The model under review builds one solid part; all positions refer to its coordinate system, in mm. A direction names the side the tool comes from. Coordinates: 2 decimals unless noted, no trailing zeros. Write each loop counter-clockwise with the first axis right and the second up, starting at its lowest first coordinate (ties: lowest second). Pieces come first, ordered by that corner, then holes.
1) For P1, Ø6, axis at x = 30, y = -4, coming from the +Z side; P2, Ø6, axis at y = 22.5, z = 0, coming from the +X side; P3, Ø5, axis at x = 156, z = 17, coming from the +Y side, all flat-tipped, find the tip position at first contact; note any pin that passes through.
2) Mouldability with a two-part tool opening along X and no side actions: class faces 5 (the flat face through (144.6, -13, -13)), 6 (the cylindrical face through (194, -20, 0)), 7 (the flat face through (149.6, 13, -13)) as released by +X, released by -X, zero draft, split by the parting line, or undercut.
3) Machinability: for faces 1 (the flat face through (3, 16, -5)), 2 (the cylindrical face through (203, -2.17, 9.76)), 3 (the cylindrical face through (1.986, -13.887, 10.648)), 4 (the flat face through (27, 0, -12.5)), which of the approach directions +Z, -Z, +X, -X, +Y, -Y give a long, thin tool a straight path to every point of the face, cutting with its end or side? Answer none if there is none.
4) Add section C-C, the plane x = 88.5. State the section outline as (y, z) points, then the cut area to 3 significant figures.
5) Add section A-A, the plane z = 0. Give the number of separate pieces and of enclosed holes in the cut face, then the cut area to 3 significant figures.
6) For line 1 (Y direction, x = 196, z = 0); line 2 (X direction, y = -20, z = 11); line 3 (X direction, y = -22.5, z = -11), list the stretches that pass through material, from the lowest coordinate up.
from build123d import *

# Parameters (mm, degrees)
OTW_R_GWINTOWANY_M63_D     = 5
OTW_R_GWINTOWANY_M63_DEPTH = 10
SFAZOWANIE1_SIZE           = 1
ZAOKR_GLENIE1_R            = 0.5
SFAZOWANIE2_SIZE           = 0.5
ZAOKR_GLENIE2_R            = 0.5
WYTNIJ_WYCI_GNI_CIE1_DEPTH = 5


with BuildPart() as part:
    # Szkic1 → Obrót1 (revolve)
    with BuildSketch(Plane.XY):
        Polygon((0, 0), (207.5, 0), (207.5, 10), (199.1, 10), (199.1, 30), (189.1, 30), (189.1, 17.5), (149.6, 17.5), (149.6, 25), (144.6, 25), (144.6, 17.5), (4.6, 17.5), (4.6, 16.5), (3, 16.5), (3, 17.5), (0, 17.5), align=None)
    revolve(axis=Axis((0, 0, 0), (-1, 0, 0)))

    # Otwór gwintowany M63
    with Locations(Plane(origin=(199.1, 0, 0), x_dir=(0, 0, -1), z_dir=(1, 0, 0))):
        with Locations((0, 22.5), (22.5, 0), (0, -22.5), (-22.5, 0)):
            Hole(OTW_R_GWINTOWANY_M63_D / 2, depth=OTW_R_GWINTOWANY_M63_DEPTH)

    # Sfazowanie1
    sfazowanie1_edges = [part.edges().sort_by_distance(p)[0] for p in [
        (207.5, -10, 0),
        (0, -17.5, 0),
    ]]
    chamfer(sfazowanie1_edges, length=SFAZOWANIE1_SIZE)

    # Zaokrąglenie1
    zaokr_glenie1_edges = [part.edges().sort_by_distance(p)[0] for p in [
        (189.1, -17.5, 0),
        (149.6, -17.5, 0),
        (144.6, -17.5, 0),
    ]]
    fillet(zaokr_glenie1_edges, radius=ZAOKR_GLENIE1_R)

    # Sfazowanie2
    sfazowanie2_edges = [part.edges().sort_by_distance(p)[0] for p in [
        (199.1, -30, 0),
        (189.1, -30, 0),
        (149.6, -25, 0),
        (144.6, -25, 0),
    ]]
    chamfer(sfazowanie2_edges, length=SFAZOWANIE2_SIZE)

    # Zaokrąglenie2
    zaokr_glenie2_edges = [part.edges().sort_by_distance(p)[0] for p in [
        (199.1, -10, 0),
    ]]
    fillet(zaokr_glenie2_edges, radius=ZAOKR_GLENIE2_R)

    # Szkic7 → Wytnij-wyciągnięcie1 (cut)
    with BuildSketch(Plane(origin=(0, 0, -17.5), x_dir=(-1, 0, 0), z_dir=(0, 0, -1))):
        with BuildLine():
            Line((-12.1, -5), (-42.1, -5))
            ThreePointArc((-42.1, -5), (-47.1, 0), (-42.1, 5))
            Line((-42.1, 5), (-12.1, 5))
            ThreePointArc((-12.1, 5), (-7.1, 0), (-12.1, -5))
        make_face()
    extrude(amount=-WYTNIJ_WYCI_GNI_CIE1_DEPTH, mode=Mode.SUBTRACT)


solid = part.part
Geometry results:
1. P1: stops at z = 17.47
1. P2: stops at x = 199.1
1. P3: stops at y = 9.8
2. face 5: released by -X
2. face 6: zero draft
2. face 7: undercut
3. face 1: none
3. face 2: +X
3. face 3: -X
3. face 4: -Z
4. outline: circle Ø35 at (0, 0)
4. area: 962 mm2
5. separate pieces: 3
5. enclosed holes: 0
5. area: 7,360 mm2
6. line 1: y = -30 to -25, -20 to 20, 25 to 30
6. line 2: x = 144.6 to 149.6, 189.1 to 199.1
6. line 3: x = 189.1 to 199.1
